from build123d import *

# Parameters (mm, degrees)
SKETCH_1_R          = 30
EXTRUDE_1_DEPTH     = 30
SKETCH_3_R          = 7.5
EXTRUDE_2_DEPTH     = 55
SKETCH_4_R          = 25
CUT_EXTRUDE_2_DEPTH = 25


with BuildPart() as part:
    # 草图1 → 凸台-拉伸1 (new body)
    with BuildSketch(Plane.XY):
        Circle(SKETCH_1_R)
    extrude(amount=EXTRUDE_1_DEPTH)

    # 草图3 → 凸台-拉伸2 (add)
    with BuildSketch(Plane(origin=(0, 0, 0), x_dir=(1, 0, 0), z_dir=(0, 1, 0))):
        with Locations((0, -12.5)):
            Circle(SKETCH_3_R)
    extrude(amount=EXTRUDE_2_DEPTH)

    # 草图4 → 切除-拉伸2 (cut)
    with BuildSketch(Plane.XY.offset(30)):
        Circle(SKETCH_4_R)
    extrude(amount=-CUT_EXTRUDE_2_DEPTH, mode=Mode.SUBTRACT)


solid = part.part
Verification items for the finished model (mm, model axes). A direction names the side the tool comes from. Round coordinates to 2 decimals unless told otherwise and drop trailing zeros. Loops run counter-clockwise (first coordinate to the right, second up) from the corner with the lowest first, then second, coordinate; pieces in that order, holes last. Notation, with made-up numbers: (82, 60) - (88, 60) arc R15 ccw to (88, 80) - close; hole circle Ø2 at (30, 19.25). An arc over 180 degrees is marked (long way). Use a Markdown table: item, result. Add a question column.
1. Access from +Z, -Z, +X, -X, +Y, -Y to the whole of each face (thin tool, end or side, straight path). Record for faces 1 (the face through (-7, 25, 30)), 2 (the face through (-1.63, 41.84, 19.82)).
2. Section check B-B, the plane x = 0. Record the boundary of the cut face in (y, z), plus the area to 3 significant figures.
3. Section check D-D, the plane x = 23.5. Record the boundary of the cut face in (y, z), plus the area to 3 significant figures.
4. Gauge pin test, flat ends, axial feed: pin 1 (1 mm diameter, centred on x = 8, z = 26.5, fed in from -Y); pin 2 (1 mm diameter, centred on x = 5.5, z = 25, fed in from -Y); pin 3 (2 mm diameter, centred on x = -12, z = 13, fed in from +Y). Record the tip position at first contact, or that the pin passes through.
5. Section check A-A, the plane z = 12.5. Record the boundary of the cut face in (x, y), plus the area to 3 significant figures.
6. Thickness scan on probe 1 along Y at (x, z) = (0, 12); probe 2 along Z at (x, y) = (-21, -3.5); probe 3 along Y at (x, z) = (10, 6). Record the ranges inside material, lowest first. Write a range as [from, to].
7. Section check C-C, the plane y = 0. Record the boundary of the cut face in (x, z), plus the area to 3 significant figures.
8. Release check for a two-part mould opening along X. For faces 3 (the face through (23.846, 7.509, 17.675)), 4 (the face through (0, 55, 12)), 5 (the face through (0, 0, 5)), 6 (the face through (-6.503, -29.287, 14.79)) record: released by +X, released by -X, zero draft, split by the parting line, or undercut.
Checks:
| question | item | result |
|---|---|---|
| 1 | face 1 | +Z, +X, -X, +Y, -Y |
| 1 | face 2 | +Y |
| 2 | outline | (-30, 0) - (30, 0) - (30, 5) - (55, 5) - (55, 20) - (30, 20) - (30, 30) - (25, 30) - (25, 5) - (-25, 5) - (-25, 30) - (-30, 30) - close |
| 2 | area | 925 mm^2 |
| 3 | outline | (-18.65, 0) - (18.65, 0) - (18.65, 30) - (8.53, 30) - (8.53, 5) - (-8.53, 5) - (-8.53, 30) - (-18.65, 30) - close |
| 3 | area | 692 mm^2 |
| 4 | pin 1 | stops at y = -29.05 |
| 4 | pin 2 | stops at y = -29.58 |
| 4 | pin 3 | stops at y = 27.91 |
| 5 | outline | (-7.5, 29.05) arc R30 ccw (long way) to (7.5, 29.05) - (7.5, 55) - (-7.5, 55) - close; hole circle Ø50 at (0, 0) |
| 5 | area | 1,240 mm^2 |
| 6 | probe 1 | y = [-30, -25], [25, 55] |
| 6 | probe 2 | z = [0, 5] |
| 6 | probe 3 | y = [-28.28, -22.91], [22.91, 28.28] |
| 7 | outline | (-30, 0) - (30, 0) - (30, 30) - (25, 30) - (25, 5) - (-25, 5) - (-25, 30) - (-30, 30) - close |
| 7 | area | 550 mm^2 |
| 8 | face 3 | undercut |
| 8 | face 4 | zero draft |
| 8 | face 5 | undercut |
| 8 | face 6 | split by the parting line |
